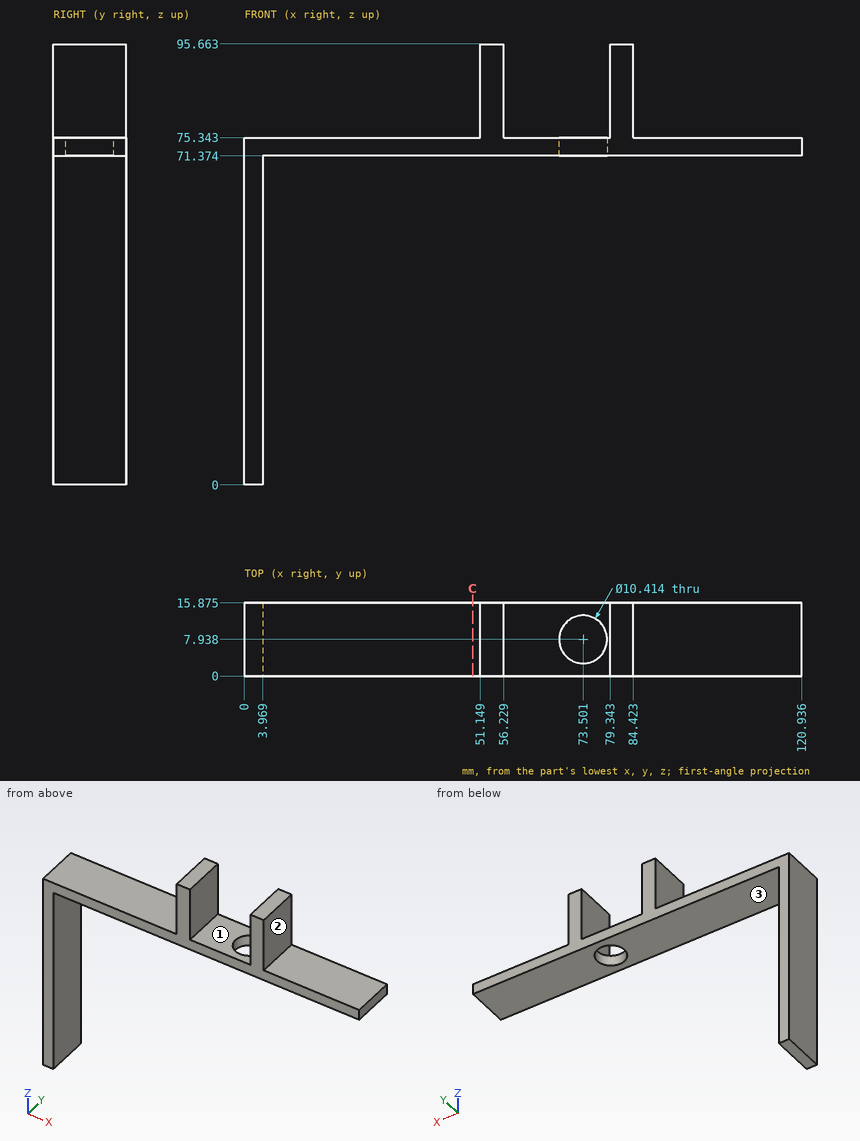
Could you check a few things on this drawing? It's one solid part, dimensions in mm from its lowest x, y, z. A direction names the side the tool comes from. Round coordinates to 2 decimals unless told otherwise and drop trailing zeros. Order: outer loops, then holes, each group sorted by start corner. A loop starts at its lowest first (then second) coordinate and runs counter-clockwise, first axis right, second up. Notation, with made-up numbers: M -26.5,51.25 L -10.5,51.25 A31 cw -10.5,87.25 Z; hole C -5,0 d11. An arc over 180 degrees is marked long. One line per item, written item: value.
(1) I need wall thicknesses on line 1 along X through (y, z) = (6.25, 64.5); line 2 along Z through (x, y) = (102, 10.5) (1 decimal); line 3 along X through (y, z) = (7.5, 80.5). Which ranges of each line are inside material? Lowest first, please. Write a range as from..to.
Ans:
line 1: x = 0..3.97
line 2: z = 71.4..75.3
line 3: x = 51.15..56.23, 79.34..84.42
(2) Which directions (+Z, -Z, +X, -X, +Y, -Y) give clear straight access to the entire face, cutting with the end or side of a thin tool? Please do the marked faces 1, 2 and 3.
Ans:
face 1: +Z, +Y, -Y
face 2: +Z, +X, +Y, -Y
face 3: -Z, +X, +Y, -Y
(3) Imagine slicing it at C-C (x = 49.5). Write out the boundary of the cut face in (y, z) (1 decimal).
Ans:
outline: M 0,71.4 L 15.9,71.4 L 15.9,75.3 L 0,75.3 Z
(4) I'm going to push flat-ended pins straight in: P1, Ø5, axis at y = 9, z = 87.5, coming from the -X side; P2, Ø5, axis at x = 87.5, y = 2, coming from the -Z side; P3, Ø8, axis at x = 14.5, y = 9.5, coming from the +Z side. Where does each tip first touch, or does it pass through?
Ans:
P1: stops at x = 51.15
P2: stops at z = 71.37
P3: stops at z = 75.34
